CAD build for the part. Positions are in the model's coordinates, mm. A direction names the side the tool comes from. Give positions to 0.01 mm unless a question says otherwise; leave off trailing zeros. Loops run counter-clockwise (first coordinate to the right, second up) from the corner with the lowest first, then second, coordinate; pieces in that order, holes last. Notation, with made-up numbers: M 71.5,83 L 130.5,83 A17 cw 130.5,96 Z; hole C 19,50 d11. An arc over 180 degrees is marked long. Answer as CSV lines item,"result".
from build123d import *

# Parameters (mm, degrees)
F0_R     = 63.5
F0_W     = 50.8
F0_H     = 50.8
F1_DEPTH = 12.7
F2_R     = 38.1
F3_DEPTH = 57.15
F4_R     = 50.8
F5_DEPTH = 12.7
F6_W     = 50.8
F6_H     = 50.8
F7_DEPTH = 82.55
F8_R     = 6.35
F9_DEPTH = 12.7


with BuildPart() as f1:
    # F0 (on Front) → F1 (new body)
    with BuildSketch(Plane.XZ):
        Circle(F0_R)
        Rectangle(F0_W, F0_H, mode=Mode.SUBTRACT)
    extrude(amount=F1_DEPTH)

    # F2 (on Front) → F3 (join)
    with BuildSketch(Plane.XZ):
        Circle(F2_R)
    extrude(amount=F3_DEPTH)

    # F4 (on face) → F5 (join)
    with BuildSketch(Plane.XZ.offset(57.15)):
        Circle(F4_R)
    extrude(amount=F5_DEPTH)

    # F6 (on face) → F7 (cut)
    with BuildSketch(Plane(origin=(0, 0, 0), x_dir=(-1, 0, 0), z_dir=(0, 1, 0))):
        Rectangle(F6_W, F6_H)
    extrude(amount=-F7_DEPTH, mode=Mode.SUBTRACT)

    # F8 (on face) → F9 (cut)
    with BuildSketch(Plane(origin=(0, 0, 0), x_dir=(-1, 0, 0), z_dir=(0, 1, 0))):
        with Locations((0, -43.060273)):
            Circle(F8_R)
    extrude(amount=-F9_DEPTH, mode=Mode.SUBTRACT)


solid = f1.part
1) Drill centre lines: line 1 (Z direction, x = 0, y = -3.75); line 2 (X direction, y = -15.5, z = -1); line 3 (Y direction, x = 43, z = -5). Where is each one in solid material? Low to high. Write a range as from..to.
Answer below:
line 1,"z = -63.5..-49.41, -36.71..-25.4, 25.4..63.5"
line 2,"x = -38.09..-25.4, 25.4..38.09"
line 3,"y = -69.85..-57.15, -12.7..0"
2) Band-saw the part on C-C on y = -19. Give the cut face in (x, z).
Answer below:
outline,"C 0,0 d76.2; hole M -25.4,-25.4 L 25.4,-25.4 L 25.4,25.4 L -25.4,25.4 Z"
3) Mould opens along X. For faces 6 (the face through (-1, -69.85, -33)), 7 (the face through (0, -34, -25.4)), 8 (the face through (-30.235, -34.614, -23.183)) say: +X half, -X half, draft (parallel to the pull), parting line (faces both ways), or undercut.
Answer below:
face 6,"draft"
face 7,"undercut"
face 8,"parting line"
4) Band-saw the part on B-B on x = 0. Give the cut face in (y, z), and give its area (3 significant figures).
Answer below:
outline,"M -69.85,-50.8 L -57.15,-50.8 L -57.15,-38.1 L -12.7,-38.1 L -12.7,-36.71 L 0,-36.71 L 0,-25.4 L -69.85,-25.4 Z; M -69.85,25.4 L 0,25.4 L 0,63.5 L -12.7,63.5 L -12.7,38.1 L -57.15,38.1 L -57.15,50.8 L -69.85,50.8 Z; M -12.7,-63.5 L 0,-63.5 L 0,-49.41 L -12.7,-49.41 Z"
area,"2,580 mm^2"
5) Which spindle directions (+Z, -Z, +X, -X, +Y, -Y) get a long thin tool onto all of the face, cutting with end or side? Do faces 1 (the face through (1.38, -6.26, -49.26)), 2 (the face through (27, 0, 1)), 3 (the face through (0, -34, 25.4)), 4 (the face through (27.3, -12.7, -27.3)), 5 (the face through (-11.012, -63.411, -49.592)). Say none if no direction does.
Answer below:
face 1,"+Y"
face 2,"+Z, -Z, +X, -X, +Y"
face 3,"+Y, -Y"
face 4,"none"
face 5,"-Y"
6) Flat gauge pins, fed straight in: pin 1 (10 mm diameter, centred on x = 41, z = -47, fed in from -Y); pin 2 (15 mm diameter, centred on x = -6.5, y = -41, fed in from +Z); pin 3 (5 mm diameter, centred on y = -54.5, z = 12, fed in from -X). Where does each tip first touch, or does it go through?
Answer below:
pin 1,"stops at y = -12.7"
pin 2,"stops at z = 38.1"
pin 3,"stops at x = -36.9"
7) Band-saw the part on A-A on z = 0. Give the cut face in (x, y).
Answer below:
outline,"M -63.5,-12.7 L -38.1,-12.7 L -38.1,-57.15 L -50.8,-57.15 L -50.8,-69.85 L -25.4,-69.85 L -25.4,0 L -63.5,0 Z; M 25.4,-69.85 L 50.8,-69.85 L 50.8,-57.15 L 38.1,-57.15 L 38.1,-12.7 L 63.5,-12.7 L 63.5,0 L 25.4,0 Z"
8) Band-saw the part on D-D on x = 45. Give the cut face in (y, z), and give its area (3 significant figures).
Answer below:
outline,"M -69.85,-23.57 L -57.15,-23.57 L -57.15,23.57 L -69.85,23.57 Z; M -12.7,-44.8 L 0,-44.8 L 0,44.8 L -12.7,44.8 Z"
area,"1,740 mm^2"
